```python
from build123d import *

# Parameters (mm, degrees)
F0_W     = 42
F0_H     = 42
F0_R     = 1.5
F1_DEPTH = 48
F2_SIZE  = 5.08
F3_R     = 11
F4_DEPTH = 2
F5_R     = 2.5
F6_DEPTH = 22


with BuildPart() as f1:
    # F0 (on Front) → F1 (new body)
    with BuildSketch(Plane.XZ):
        Rectangle(F0_W, F0_H)
        with Locations((-15.67623, -15.695493)):
            Circle(F0_R, mode=Mode.SUBTRACT)
        with Locations((15.32377, -15.667882)):
            Circle(F0_R, mode=Mode.SUBTRACT)
        with Locations((-15.472639, 15.304507)):
            Circle(F0_R, mode=Mode.SUBTRACT)
        with Locations((15.527361, 15.332118)):
            Circle(F0_R, mode=Mode.SUBTRACT)
    extrude(amount=F1_DEPTH)

    # F2
    f2_edges = [f1.edges().sort_by_distance(p)[0] for p in [
        (-21, -24, 21),
        (21, -24, 21),
        (21, -24, -21),
        (-21, -24, -21),
    ]]
    chamfer(f2_edges, length=F2_SIZE)

    # F3 (on face) → F4 (join)
    with BuildSketch(Plane.XZ.offset(48)):
        Circle(F3_R)
    extrude(amount=F4_DEPTH)

    # F5 (on face) → F6 (join)
    with BuildSketch(Plane.XZ.offset(50)):
        Circle(F5_R)
    extrude(amount=F6_DEPTH)


solid = f1.part
```
Geometry: final body of the model. Coordinates: model frame, mm. A direction names the side the tool comes from. Round coordinates to 2 decimals unless told otherwise and drop trailing zeros. Order: outer loops, then holes, each group sorted by start corner. A loop starts at its lowest first (then second) coordinate and runs counter-clockwise, first axis right, second up. Notation, with made-up numbers: M 48,76.5 L 79,76.5 A8 cw 79,83.5 Z; hole C -4,18.25 d11. An arc over 180 degrees is marked long. One line per item, written item: value.
(1) Cut plane C-C (z = 0). Return the cut outline in (x, y).
Result sheet:
outline: M -21,-48 L -11,-48 L -11,-50 L -2.5,-50 L -2.5,-72 L 2.5,-72 L 2.5,-50 L 11,-50 L 11,-48 L 21,-48 L 21,0 L -21,0 Z
(2) Cut plane D-D (z = -7). Return the cut outline in (x, y).
Result sheet:
outline: M -21,-48 L -8.49,-48 L -8.49,-50 L 8.49,-50 L 8.49,-48 L 21,-48 L 21,0 L -21,0 Z
(3) Cut plane A-A (y = -37). Return the cut outline in (x, z), and give its area (3 significant figures).
Result sheet:
outline: M -21,-15.92 L -15.92,-21 L 15.92,-21 L 21,-15.92 L 21,15.92 L 15.92,21 L -15.92,21 L -21,15.92 Z; hole C -15.68,-15.7 d3; hole C -15.47,15.3 d3; hole C 15.32,-15.67 d3; hole C 15.53,15.33 d3
area: 1,680 mm2
(4) Pin query (flat end, axial travel): P1, Ø5, axis at x = -15.47, z = 15.3, coming from the -Y side; P2, Ø3, axis at x = 6.5, z = -8.5, coming from the -Y side; P3, Ø2.5, axis at x = 15.53, z = 15.33, coming from the -Y side. Return the tip coordinate at first contact, or that it passes through.
Result sheet:
P1: y = -48
P2: y = -50
P3: through
(5) Reachability of faces 4 (the flat face through (9, -48, -9)), 5 (the flat face through (-21, -24, 0)) from +Z, -Z, +X, -X, +Y, -Y: full face, straight path, thin tool, end or side. Return the list, or none.
Result sheet:
face 4: -Y
face 5: +Z, -Z, -X, +Y, -Y
(6) Cut plane B-B (x = 0). Return the cut outline in (y, z).
Result sheet:
outline: M -72,-2.5 L -50,-2.5 L -50,-11 L -48,-11 L -48,-21 L 0,-21 L 0,21 L -48,21 L -48,11 L -50,11 L -50,2.5 L -72,2.5 Z
(7) Line query: probe 1 along Z at (x, y) = (-15.5, -8.5); probe 2 along X at (y, z) = (-40, 15.5); probe 3 along Y at (x, z) = (1, -3.5). Output: solid intervals per line, ascending. Write a range as [from, to].
Result sheet:
probe 1: [-21, -17.19], [-14.21, 13.8], [16.8, 21]
probe 2: [-21, -16.96], [-13.99, 14.04], [17.02, 21]
probe 3: [-50, 0]
(8) Pull-direction query (X, two-part tool) for faces 1 (the cylindrical face through (-14.87, -23.66, -14.43)), 2 (the flat face through (18.5, -23.66, 18.42)), 3 (the cylindrical face through (-2.38, -48.99, -10.74)); classes: pulls with the +X half, pulls with the -X half, needs draft (parallel to the pull), parting line crosses it, or undercut.
Result sheet:
face 1: undercut
face 2: pulls with the +X half
face 3: parting line crosses it
